Build history of the part. All positions in model axes, mm. A direction names the side the tool comes from. Round coordinates to 2 decimals unless told otherwise and drop trailing zeros. Order: outer loops, then holes, each group sorted by start corner. A loop starts at its lowest first (then second) coordinate and runs counter-clockwise, first axis right, second up. Notation, with made-up numbers: (18.5, 44) -> (72.5, 44) arc R19 ccw to (72.5, 81) -> close; hole circle Ø9 at (63, 14). An arc over 180 degrees is marked (long way). Answer as a JSON object with one key per item and string values.
from build123d import *

# Parameters (mm, degrees)
SKETCH3_W           = 19.685
SKETCH3_H           = 19.685
BOSS_EXTRUDE2_DEPTH = 38.1
SKETCH5_R           = 2.54
CUT_EXTRUDE2_DEPTH  = 5.715
SKETCH6_W           = 10.4775
SKETCH6_H           = 10.4775
CUT_EXTRUDE3_DEPTH  = 16.51
SKETCH7_W           = 2.032
SKETCH7_H           = 4.572
SKETCH7_W_2         = 4.572
SKETCH7_H_2         = 2.032
CUT_EXTRUDE4_DEPTH  = 5.08
CHAMFER1_SIZE       = 9.525


with BuildPart() as part:
    # Sketch3 → Boss-Extrude2 (new body)
    with BuildSketch(Plane(origin=(0, 0, 0), x_dir=(1, 0, 0), z_dir=(0, 1, 0))):
        Rectangle(SKETCH3_W, SKETCH3_H)
    extrude(amount=BOSS_EXTRUDE2_DEPTH)

    # Sketch5 → Cut-Extrude2 (cut)
    with BuildSketch(Plane.XZ):
        with Locations(Location((-4.92125, 4.92125, 0), (0, 0, 270))):
            Circle(SKETCH5_R)
    extrude(amount=-CUT_EXTRUDE2_DEPTH, mode=Mode.SUBTRACT)

    # Sketch6 → Cut-Extrude3 (cut)
    with BuildSketch(Plane(origin=(0, 38.1, 0), x_dir=(1, 0, 0), z_dir=(0, 1, 0))):
        with Locations((4.60375, 4.60375)):
            Rectangle(SKETCH6_W, SKETCH6_H)
    extrude(amount=-CUT_EXTRUDE3_DEPTH, mode=Mode.SUBTRACT)

    # Sketch7 → Cut-Extrude4 (cut)
    with BuildSketch(Plane(origin=(0, 38.1, 0), x_dir=(1, 0, 0), z_dir=(0, 1, 0))):
        with Locations((-5.23875, 5.0165)):
            Rectangle(SKETCH7_W, SKETCH7_H)
        with Locations((5.0165, -5.23875)):
            Rectangle(SKETCH7_W_2, SKETCH7_H_2)
    extrude(amount=-CUT_EXTRUDE4_DEPTH, mode=Mode.SUBTRACT)

    # Chamfer1
    chamfer1_edges = [part.edges().sort_by_distance(p)[0] for p in [
        (9.8425, 10.795, -9.8425),
    ]]
    chamfer(chamfer1_edges, length=CHAMFER1_SIZE)


solid = part.part
1) Probe L1, parallel to Y at x = -5, z = -4.75; L2, parallel to Y at x = 1.25, z = -8; L3, parallel to Z at x = 5.25, y = 26.5 (1 decimal). List the from-to ranges inside material, lowest first. Write a range as from..to.
Checked values:
{"L1": "y = 0..33.02", "L2": "y = 0..21.59", "L3": "z = 0.6..9.8"}
2) Cut at C-C, the plane y = 18. Give the cut face in (x, z).
Checked values:
{"outline": "(-9.84, -9.84) -> (0.32, -9.84) -> (9.84, -0.32) -> (9.84, 9.84) -> (-9.84, 9.84) -> close"}
3) Cut at B-B, the plane z = -8. Give the cut face in (x, y) (1 decimal).
Checked values:
{"outline": "(-9.8, 0) -> (2.2, 0) -> (2.2, 21.6) -> (-0.6, 21.6) -> (-0.6, 38.1) -> (-9.8, 38.1) -> close"}
4) Cut at D-D, the plane x = 1.25. Give the cut face in (y, z) (1 decimal), plus the area to 3 significant figures.
Checked values:
{"outline": "(0, -8.9) -> (21.6, -8.9) -> (21.6, 0.6) -> (38.1, 0.6) -> (38.1, 9.8) -> (0, 9.8) -> close", "area": "557 mm²"}
5) Which spindle directions (+Z, -Z, +X, -X, +Y, -Y) get a long thin tool onto all of the face, cutting with end or side? Do faces 4 (the face through (-4.16, 2.82, 2.5)), 5 (the face through (5, 30, 0.635)), 6 (the face through (-5, 36, -7.302)). Say none if no direction does.
Checked values:
{"face 4": "-Y", "face 5": "-Z, +X, +Y", "face 6": "+Y"}
6) Flat gauge pins, fed straight in: pin 1 Ø3 at (x, y) = (4.5, 33) entering from -Z (3 decimals); pin 2 Ø3 at (y, z) = (6.5, -5) entering from +X; pin 3 Ø1 at (x, z) = (-5, -4.5) entering from +Y. Where does each tip first touch, or does it go through?
Checked values:
{"pin 1": "stops at z = 0.635", "pin 2": "stops at x = 6.66", "pin 3": "stops at y = 33.02"}
7) Cut at A-A, the plane y = 34.5. Give the cut face in (x, z) (1 decimal).
Checked values:
{"outline": "(-9.8, -9.8) -> (-0.6, -9.8) -> (-0.6, 0.6) -> (9.8, 0.6) -> (9.8, 9.8) -> (-9.8, 9.8) -> close; hole (-6.3, -7.3) -> (-4.2, -7.3) -> (-4.2, -2.7) -> (-6.3, -2.7) -> close; hole (2.7, 4.2) -> (7.3, 4.2) -> (7.3, 6.3) -> (2.7, 6.3) -> close"}
8) Pull direction Z, two halves, no side cores. Call faces 1 (the face through (3, 21.59, -4)), 2 (the face through (5.15, 10.64, -5.01)), 3 (the face through (-5, 5.715, 5)): pulls with the +Z half, pulls with the -Z half, needs draft (parallel to the pull), parting line crosses it, or undercut.
Checked values:
{"face 1": "needs draft", "face 2": "pulls with the -Z half", "face 3": "undercut"}
